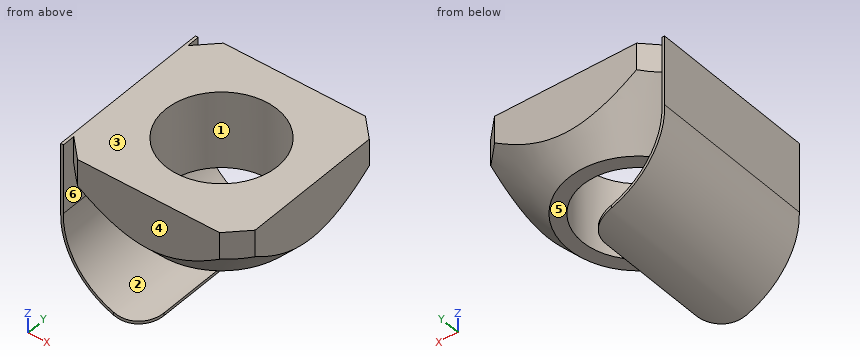
Autodesk Inventor part; units mm, degrees
ref_plane "Work Plane1" through (-5.7929, -5.7929, -5.5) normal (0.7071068, -0.7071068, 0) x (0.7071068, 0.7071068, 0)
ref_plane "YZ Plane" through (0, 0, 0) normal (1, 0, 0) x (0, 1, 0)
ref_plane "XZ Plane" through (0, 0, 0) normal (0, 1, 0) x (-1, 0, 0)
sketch "Sketch2" plane through (0, 0, 0) normal (0, 0, 1) x (1, 0, 0)
  line L0 (-5.0858, -6.5) -> (5.0858, -6.5)
  line L1 (6.5, -5.0858) -> (6.5, 5.0858)
  line L2 (5.0858, 6.5) -> (-5.0858, 6.5)
  line L3 (-6.5, 5.0858) -> (-6.5, -5.0858)
  line L4 (-6.5, 6.5) -> (6.5, -6.5) construction
  circle A0 centre (0, 0) radius 4
  line L5 (5.0858, 6.5) -> (6.5, 5.0858)
  line L6 (0, -6.5) -> (0, 6.5) construction
  line L7 (-6.5, 0) -> (6.5, 0) construction
  line L8 (-5.0858, 6.5) -> (-6.5, 5.0858)
  line L9 (5.0858, -6.5) -> (6.5, -5.0858)
  line L10 (-5.0858, -6.5) -> (-6.5, -5.0858)
  dimension "THREAD" = 8
  dimension "d3" = 45
  dimension "d4" = 2
extrude "Extrusion1" add sketch "Sketch2" against normal blind 5.5
ref_plane "Work Plane1" through (-5.7929, -5.7929, -5.5) normal (0.7071068, -0.7071068, 0) x (0.7071068, 0.7071068, 0)
sketch "Sketch4" plane through (-5.7929, -5.7929, -5.5) normal (0.7071068, -0.7071068, 0) x (0.7071068, 0.7071068, 0)
  line L0 (12.1924, 0) -> (4.1924, 0)
  line L1 (8.1924, 0) -> (13.1924, 0)
  line L2 (16.3848, 5.5) -> (16.3848, 3.5)
  line L3 (13.1924, 0) -> (16.7968, 3.9518)
  line L4 (13.1924, 0) -> (16.3848, 0)
  line L5 (16.3848, 3.5) -> (16.3848, 0)
  line L6 (16.7968, 3.9518) -> (16.7968, -0.4121)
  line L7 (16.7968, -0.4121) -> (13.1924, -0.4121)
  line L8 (13.1924, -0.4121) -> (13.1924, 0)
  line L9 (8.1924, 5.5) -> (8.1924, 0)
  line L10 (16.3848, 5.5) -> (16.3848, 0)
  line L11 (16.3848, 3.5) -> (17.5015, 3.5) construction
  line L12 (9.1924, 5.5) -> (16.3848, 5.5) construction
  dimension "d10" = 5
  dimension "d15" = 2
revolve "Revolution1" cut sketch "Sketch4" angle 360 about axis through (0, 0, 0) along (0, 0, -1)
thread "Thread1"
sketch "Sketch6" plane through (-3.5464, 0, 2.5351) normal (0, 1, 0) x (-1, 0, 0)
  line L0 (2.9536, -2.5351) -> (2.9536, 6.0056)
  line L1 (2.9536, -2.5351) -> (2.9536, -7.5351)
  arc A0 (-2.6464, -13.1351) -> (2.9536, -7.5351) centre (-2.4158, -7.7657) ccw
  line L2 (2.9536, -2.5351) -> (3.1536, -2.5351)
  line L3 (3.1536, -2.5351) -> (3.1536, -7.5351)
  line L4 (-2.6464, -13.1351) -> (-2.6464, -13.3351)
  arc A1 (-2.6464, -13.3351) -> (3.1536, -7.5351) centre (-2.4158, -7.7657) ccw
  line L5 (2.9536, 0) -> (2.9536, -1.9333)
  line L6 (-5.0858, -2.5351) -> (5.0858, -2.5351)
  line L7 (-8.6322, -2.5351) -> (1.5394, -2.5351)
  line L8 (2.9536, -2.5351) -> (2.9536, -4.4684)
  point P0 (0, 0)
  point P1 (-15.0649, 7.0019)
  dimension "d25" = 5
  dimension "d23" = 0.2
  dimension "d22" = 0.2
  dimension "d21" = 10.8
  dimension "d24" = 5.3743
extrude "Extrusion3" add sketch "Sketch6" along normal mid plane 12
fillet "Fillet2" radius 2 2 edges at (-0.9, -6, -10.7) (-0.9, 6, -10.7)
properties part number "21.1351/2" material "Steel, Mild"
Check sheet for the modelled part. Datum: model origin and axes. Units: mm. Face numbers are marked on the shaded views. A direction names the side the tool comes from. Round coordinates to 2 decimals unless told otherwise and drop trailing zeros. Order: outer loops, then holes, each group sorted by start corner. A loop starts at its lowest first (then second) coordinate and runs counter-clockwise, first axis right, second up. Notation, with made-up numbers: (-13.75, -17) -> (-3.75, -17) arc R7 ccw to (-3.75, -5) -> close; hole circle Ø11 at (66, 64). An arc over 180 degrees is marked (long way). Use CSV: the item, a comma, the result in double quotes.
(1) Material ranges on line 1 along Z through (x, y) = (-1.25, -4.75); line 2 along X through (y, z) = (0.75, -4.25); line 3 along Y through (x, z) = (0, -2.6), recorded low to high. Write a range as from..to.
Worked out:
line 1,"-10.8..-10.6, -5.5..0"
line 2,"-6.7..-6.5, -6.09..-3.93, 3.93..6.09"
line 3,"-6.5..-4, 4..6.5"
(2) Tool access check on the marked faces 4, 5 and 6. Record the directions out of +Z, -Z, +X, -X, +Y, -Y that give a thin tool (end or side, any length) a straight path to the whole face; none if there is none.
Worked out:
face 4,"+Z, -Z, +X, -X, -Y"
face 5,"+X, +Y, -Y"
face 6,"none"
(3) Cross-section at A-A (y = 0). Record the boundary of the cut face in (x, z), and give its area (3 significant figures).
Worked out:
outline,"(-6.7, -5) arc R5.57 ccw to (-0.9, -10.8) -> (-0.9, -10.6) arc R5.37 cw to (-6.5, -5) -> (-6.5, -3.86) -> (-5, -5.5) -> (-4, -5.5) -> (-4, 0) -> (-6.7, 0) -> close; (4, -5.5) -> (5, -5.5) -> (6.5, -3.86) -> (6.5, 0) -> (4, 0) -> close"
area,"27.8 mm²"
(4) Cross-section at B-B (z = -1.5). Record the boundary of the cut face in (x, y), and give its area (3 significant figures).
Worked out:
outline,"(-6.7, -6) -> (-6.5, -6) -> (-6.5, -5.09) -> (-5.09, -6.5) -> (5.09, -6.5) -> (6.5, -5.09) -> (6.5, 5.09) -> (5.09, 6.5) -> (-5.09, 6.5) -> (-6.5, 5.09) -> (-6.5, 6) -> (-6.7, 6) -> close; hole circle Ø8 at (0, 0)"
area,"117 mm²"
(5) Depth check by flat-ended pin: pin 1 (6.5 mm diameter, centred on x = 0, y = 0, fed in from +Z); pin 2 (1.9 mm diameter, centred on x = -5.5, z = -3, fed in from +Y); pin 3 (1.5 mm diameter, centred on y = 5, z = -6.5, fed in from +X). Enter the tip coordinate at first touch or a pass-through.
Worked out:
pin 1,"z = -10.17"
pin 2,"y = 6.27"
pin 3,"x = -6.11"
(6) Cross-section at C-C (x = 0). Record the boundary of the cut face in (y, z).
Worked out:
outline,"(-6.5, -3.86) -> (-5, -5.5) -> (-4, -5.5) -> (-4, 0) -> (-6.5, 0) -> close; (4, -5.5) -> (5, -5.5) -> (6.5, -3.86) -> (6.5, 0) -> (4, 0) -> close"
(7) Draft check along Z on the marked faces 1, 2 and 3. Enter one of: pulls with the +Z half, pulls with the -Z half, needs draft (parallel to the pull), parting line crosses it, or undercut.
Worked out:
face 1,"needs draft"
face 2,"undercut"
face 3,"pulls with the +Z half"
(8) Cross-section at D-D (z = -3.5). Record the boundary of the cut face in (x, y), and give its area (3 significant figures).
Worked out:
outline,"(-6.7, -6) -> (-6.5, -6) -> (-6.5, -2.08) arc R6.82 ccw to (-2.08, -6.5) -> (2.08, -6.5) arc R6.82 ccw to (6.5, -2.08) -> (6.5, 2.08) arc R6.82 ccw to (2.08, 6.5) -> (-2.08, 6.5) arc R6.82 ccw to (-6.5, 2.08) -> (-6.5, 6) -> (-6.7, 6) -> close; hole circle Ø8 at (0, 0)"
area,"94.8 mm²"
